Can you work these out from the model? Positions are in its coordinate system, mm. Face numbers are marked on the shaded views. A direction names the side the tool comes from. Round coordinates to 2 decimals unless told otherwise and drop trailing zeros. Write each loop counter-clockwise with the first axis right and the second up, starting at its lowest first coordinate (ties: lowest second). Pieces come first, ordered by that corner, then holes.
Q1. If we section it at B-B (z = 0): Please give me the cut outline in (x, y), plus the area to 3 significant figures.
Q2. For the marked faces 1, 2 and 3, which set-ups out of +Z, -Z, +X, -X, +Y, -Y let a thin tool reach every point of the face, with its end or its side?
Q3. If we section it at A-A (x = -50): Please give me the cut outline in (y, z), plus the area to 3 significant figures.
Q4. If we section it at D-D (z = 13): Please give me the cut outline in (x, y), plus the area to 3 significant figures.
Q5. Please list where these lines run through material, in increasing order: line 1 along X through (y, z) = (11.25, 0); line 2 along X through (y, z) = (1.5, -0.5); line 3 along Z through (x, y) = (-50, 8.25).
Q6. I'm going to push flat-ended pins straight in: pin 1 Ø6 at (x, z) = (53.5, 6.5) entering from -Y; pin 2 Ø1.5 at (x, z) = (3.5, -1) entering from +Y; pin 3 Ø5 at (x, z) = (0.5, 11.5) entering from +Y. Where does each tip first touch, or does it pass through?
Q7. We'd pull the mould along X, two halves only. Please class the marked faces 4, 5, 6 and 7: +X half, -X half, draft (parallel to the pull), parting line (faces both ways), or undercut.
Q8. If we section it at C-C (y = 12.5): Please give me the cut outline in (x, z).
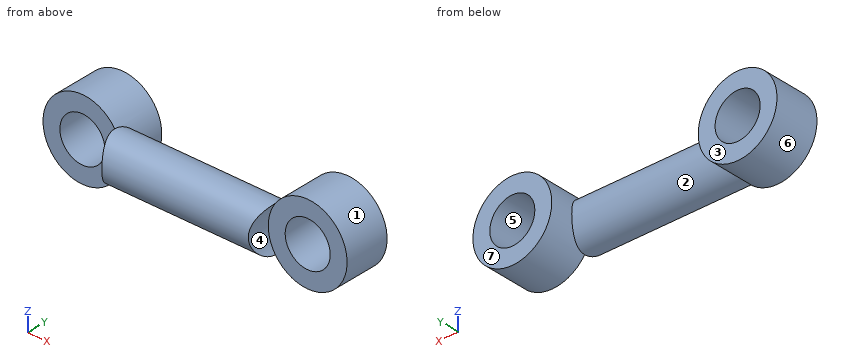
Autodesk Inventor part; units mm, degrees
ref_plane "YZ Plane" through (0, 0, 0) normal (1, 0, 0) x (0, 1, 0)
ref_plane "XZ Plane" through (0, 0, 0) normal (0, 1, 0) x (-1, 0, 0)
ref_plane "XY Plane" through (0, 0, 0) normal (0, 0, 1) x (1, 0, 0)
sketch "Sketch1" plane through (0, 0, 0) normal (0, 0, 1) x (1, 0, 0)
  line L0 (-50, 0) -> (50, 0)
  line L1 (0, 0) -> (0, 34.9563) construction
  line L2 (-50, 0) -> (-50, 10)
  line L3 (-50, 10) -> (50, 10)
  line L4 (50, 10) -> (50, 0)
  dimension "d0" = 100
  dimension "d1" = 10
revolve "Revolution1" add sketch "Sketch1" angle 360 about axis through (-50, 0, 0) along (1, 0, 0)
sketch "Sketch2" plane through (0, 0, 0) normal (0, 1, 0) x (-1, 0, 0)
  line L0 (-50, 10) -> (-50, -10)
  circle A0 centre (-50, 0) radius 17.5
  circle A1 centre (-50, 0) radius 10
  point P0 (0, 0)
  dimension "d3" = 35
  dimension "d4" = 20
extrude "Extrusion1" add sketch "Sketch2" along normal blind 20
extrude "Extrusion2" cut sketch "Sketch2" against normal blind 20 contours A1 L0 | A0 picked at (-47.9217, -2.6061)
extrude "Extrusion3" cut sketch "Sketch2" along normal blind 20 contours A1 L0 picked at (-47.9217, -2.6061)
sketch "Sketch4" plane through (0, 0, 0) normal (0, 1, 0) x (-1, 0, 0)
  line L0 (50, 10) -> (50, -10)
  circle A0 centre (50, 0) radius 17.5
  circle A1 centre (50, 0) radius 10
  point P0 (0, 0)
  dimension "d17" = 35
  dimension "d18" = 20
extrude "Extrusion6" add sketch "Sketch4" along normal blind 20
extrude "Extrusion7" cut sketch "Sketch4" against normal blind 20 contours L0 A1 | A0 picked at (46.9919, -2.3982)
extrude "Extrusion8" cut sketch "Sketch4" along normal blind 20 contours L0 A1 picked at (46.9919, -2.3982)
A:
1. outline: (-67.5, 0) - (-60, 0) - (-60, 20) - (-67.5, 20) - close; (-40, 0) - (-32.5, 0) - (-32.5, -10) - (32.5, -10) - (32.5, 0) - (40, 0) - (40, 20) - (32.5, 20) - (32.5, 10) - (-32.5, 10) - (-32.5, 20) - (-40, 20) - close; (60, 0) - (67.5, 0) - (67.5, 20) - (60, 20) - close
1. area: 1,900 mm2
2. face 1: +Y
2. face 2: none
2. face 3: +Z, -Z, +X, -X, +Y
3. outline: (0, -17.5) - (20, -17.5) - (20, -10) - (0, -10) - close; (0, 10) - (20, 10) - (20, 17.5) - (0, 17.5) - close
3. area: 300 mm2
4. outline: (-61.72, 0) - (-38.28, 0) - (-38.28, 20) - (-61.72, 20) - close; (38.28, 0) - (61.72, 0) - (61.72, 20) - (38.28, 20) - close
4. area: 937 mm2
5. line 1: x = -67.5 to -60, -40 to -32.5, 32.5 to 40, 60 to 67.5
5. line 2: x = -67.49 to -59.99, -40.01 to 40.01, 59.99 to 67.49
5. line 3: z = -17.5 to -10, 10 to 17.5
6. pin 1: stops at y = 0
6. pin 2: stops at y = 10
6. pin 3: stops at y = 4.36
7. face 4: +X half
7. face 5: undercut
7. face 6: undercut
7. face 7: draft
8. outline: circle Ø35 at (-50, 0); circle Ø35 at (50, 0); hole circle Ø20 at (-50, 0); hole circle Ø20 at (50, 0)
